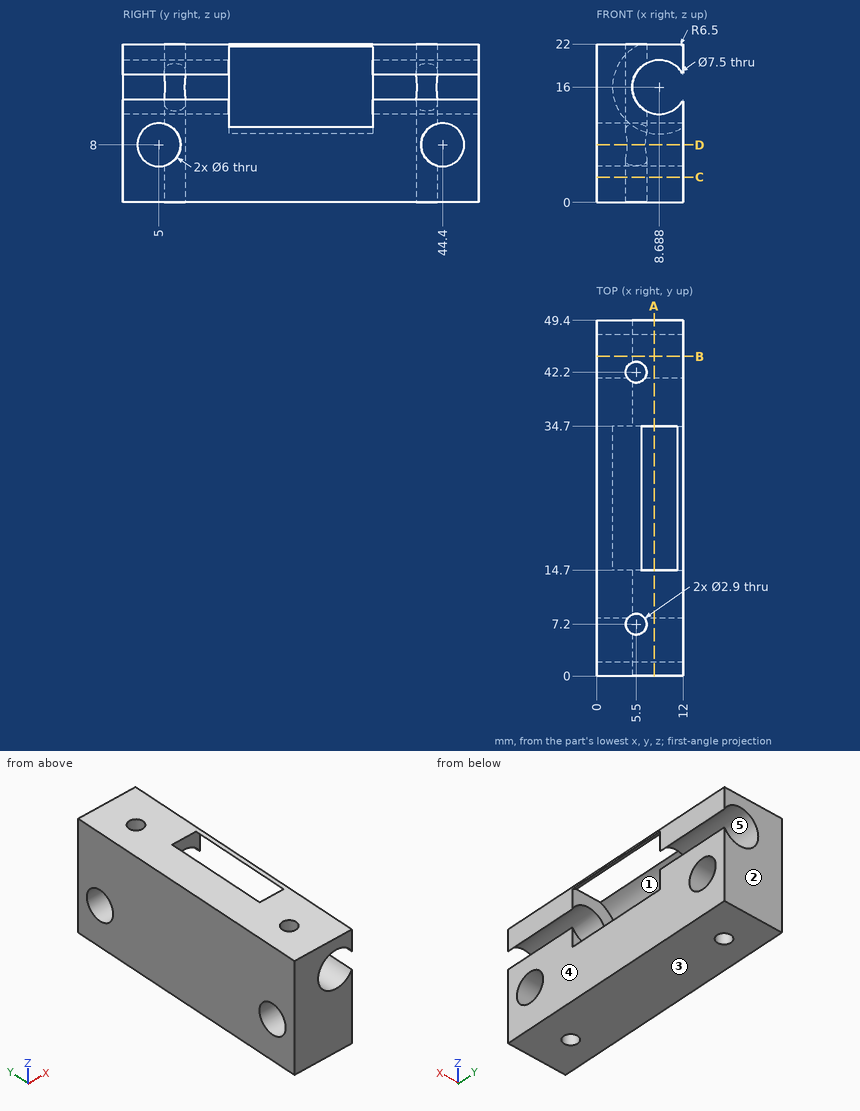
Drawing for the job (mm, zero at the part's lowest x, y, z). A direction names the side the tool comes from. Round coordinates to 2 decimals unless told otherwise and drop trailing zeros. Write each loop counter-clockwise with the first axis right and the second up, starting at its lowest first coordinate (ties: lowest second). Pieces come first, ordered by that corner, then holes. Notation, with made-up numbers: M -28.5,73 L 19.5,73 A23 ccw 19.5,96 Z; hole C 65,-39 d2. An arc over 180 degrees is marked long. Answer as a JSON object with one key per item and string values. Group by question number.
(1) Cut at C-C (z = 3.5). Give the cut face in (x, y), and give its area (3 significant figures).
(2) Cut at A-A (x = 8). Give the cut face in (y, z), and give its area (3 significant figures).
(3) Cut at B-B (y = 44.4). Give the cut face in (x, z).
(4) Drill centre lines: L1, parallel to Y at x = 5.5, z = 12.75; L2, parallel to Y at x = 10.25, z = 20.5; L3, parallel to Y at x = 5.5, z = 6.5. Where is each one in solid material? Low to high.
(5) Which spindle directions (+Z, -Z, +X, -X, +Y, -Y) get a long thin tool onto all of the face, cutting with end or side? Do the marked faces 1 and 2. Say none if no direction does.
(6) Cut at D-D (z = 8). Give the cut face in (x, y), and give its area (3 significant figures).
(7) Mould opens along X. For the marked faces 3, 4 and 5 say: pulls with the +X half, pulls with the -X half, needs draft (parallel to the pull), parting line crosses it, or undercut.
Responses:
{
 "1": {"outline": "M 0,0 L 12,0 L 12,49.4 L 0,49.4 Z; hole C 5.5,7.2 d2.9; hole C 5.5,42.2 d2.9", "area": "580 mm2"},
 "2": {"outline": "M 0,0 L 49.4,0 L 49.4,12.31 L 34.7,12.31 L 34.7,9.54 L 14.7,9.54 L 14.7,12.31 L 0,12.31 Z; M 0,19.69 L 14.7,19.69 L 14.7,22 L 0,22 Z; M 34.7,19.69 L 49.4,19.69 L 49.4,22 L 34.7,22 Z; hole C 5,8 d6; hole C 44.4,8 d6", "area": "564 mm2"},
 "3": {"outline": "M 0,0 L 12,0 L 12,5 L 0,5 Z; M 0,11 L 12,11 L 12,14.24 A3.75 cw long 12,17.76 L 12,22 L 0,22 Z"},
 "4": {"L1": "y = 0 to 5.75, 8.65 to 14.7, 34.7 to 40.75, 43.65 to 49.4", "L2": "y = 0 to 14.7, 34.7 to 49.4", "L3": "y = 0 to 2.4, 8.65 to 40.75, 47 to 49.4"},
 "5": {"face 1": "none", "face 2": "+Z, -Z, +X, -X, +Y"},
 "6": {"outline": "M 0,0 L 12,0 L 12,2 L 0,2 Z; M 0,8 L 4.29,8 A1.45 cw 6.71,8 L 12,8 L 12,41.4 L 6.71,41.4 A1.45 cw 4.29,41.4 L 0,41.4 Z; M 0,47.4 L 12,47.4 L 12,49.4 L 0,49.4 Z", "area": "447 mm2"},
 "7": {"face 3": "needs draft", "face 4": "pulls with the +X half", "face 5": "undercut"}
}
